```python
from build123d import *

# Parameters (mm, degrees)
ESQUISSE1_R                  = 5
ESQUISSE1_R_2                = 4
BOSS_EXTRU_1_DEPTH           = 15
BOSS_EXTRU_2_START           = 1.5
ESQUISSE2_R                  = 11
ESQUISSE2_R_2                = 5
BOSS_EXTRU_2_DEPTH           = 3.5
ESQUISSE3_R                  = 2
ENL_V_MAT_EXTRU_1_DEPTH      = 22.610182785
R_P_TITION_CIRCULAIRE1_COUNT = 4


with BuildPart() as part:
    # Esquisse1 → Boss.-Extru.1 (new body)
    with BuildSketch(Plane.XY):
        Circle(ESQUISSE1_R)
        Circle(ESQUISSE1_R_2, mode=Mode.SUBTRACT)
    extrude(amount=BOSS_EXTRU_1_DEPTH)

    # Esquisse2 → Boss.-Extru.2 (add)
    with BuildSketch(Plane.XY.offset(BOSS_EXTRU_2_START)):
        Circle(ESQUISSE2_R)
        Circle(ESQUISSE2_R_2, mode=Mode.SUBTRACT)
    extrude(amount=BOSS_EXTRU_2_DEPTH)

    # Esquisse3 → Enlèv. mat.-Extru.1 (cut, through all)
    with BuildSketch(Plane.XY):
        with Locations((0, 8)):
            Circle(ESQUISSE3_R)
    enl_v_mat_extru_1 = extrude(amount=ENL_V_MAT_EXTRU_1_DEPTH, mode=Mode.SUBTRACT)

    # Répétition circulaire1: Enlèv. mat.-Extru.1 ×4 about axis
    r_p_tition_circulaire1_axis = Axis((0, 0, 0), (0, 0, 1))
    for i in range(1, R_P_TITION_CIRCULAIRE1_COUNT):
        add(enl_v_mat_extru_1.rotate(r_p_tition_circulaire1_axis, i * 360 / R_P_TITION_CIRCULAIRE1_COUNT), mode=Mode.SUBTRACT)


solid = part.part
```
Geometry: final body of the model. Coordinates: model frame, mm. A direction names the side the tool comes from. Give positions to 0.01 mm unless a question says otherwise; leave off trailing zeros. Order: outer loops, then holes, each group sorted by start corner. A loop starts at its lowest first (then second) coordinate and runs counter-clockwise, first axis right, second up. Notation, with made-up numbers: (-28.5, -11) -> (5.5, -11) arc R18 cw to (5.5, 6) -> close; hole circle Ø8 at (-9, -34). An arc over 180 degrees is marked (long way). Write each question's results on one line, items separated by ' | '. Start each with the question number.
1) Section D-D (y = 6.5). Return loops of the section in (x, z).
2) Section A-A (y = 0). Return loops of the section in (x, z).
3) Section C-C (z = 3.5). Return loops of the section in (x, y).
4) Set-up query: faces 1 (the cylindrical face through (0, -10, 3)), 2 (the cylindrical face through (-1.08, -4.88, 9.93)), 3 (the flat face through (5, -2, 1.5)). Return all of +Z, -Z, +X, -X, +Y, -Y with unobstructed straight access to the full face (end or side cutting, diameter ignored); none if empty.
5) Draft query along Y for faces 4 (the flat face through (5, -2, 5)), 5 (the cylindrical face through (-1.08, -4.88, 0.74)), 6 (the cylindrical face through (10, 0, 3)). Return one class per face: pulls with the +Y half, pulls with the -Y half, needs draft (parallel to the pull), parting line crosses it, or undercut.
6) First-contact query: pin 1 (8 mm diameter, centred on y = -3.5, z = 10.5, fed in from +X); pin 2 (4 mm diameter, centred on x = 5, z = 9.5, fed in from +Y); pin 3 (4.5 mm diameter, centred on x = 8, y = 0, fed in from +Z). Flat tips, straight axial feed; report the tip coordinate or a pass-through.
7) Line query: line 1 (Y direction, x = 0, z = 3.9); line 2 (X direction, y = -1, z = 1.75); line 3 (Z direction, x = 2.5, y = 9.25). Output: solid intervals per line, ascending. Write a range as from..to.
Calculated:
1) outline: (-8.87, 1.5) -> (-1.32, 1.5) -> (-1.32, 5) -> (-8.87, 5) -> close; (1.32, 1.5) -> (8.87, 1.5) -> (8.87, 5) -> (1.32, 5) -> close
2) outline: (-11, 1.5) -> (-10, 1.5) -> (-10, 5) -> (-11, 5) -> close; (-6, 1.5) -> (-5, 1.5) -> (-5, 0) -> (-4, 0) -> (-4, 15) -> (-5, 15) -> (-5, 5) -> (-6, 5) -> close; (4, 0) -> (5, 0) -> (5, 1.5) -> (6, 1.5) -> (6, 5) -> (5, 5) -> (5, 15) -> (4, 15) -> close; (10, 1.5) -> (11, 1.5) -> (11, 5) -> (10, 5) -> close
3) outline: circle Ø22 at (0, 0); hole circle Ø4 at (-8, 0); hole circle Ø8 at (0, 0); hole circle Ø4 at (0, -8); hole circle Ø4 at (0, 8); hole circle Ø4 at (8, 0)
4) face 1: +Z, -Z | face 2: +Z | face 3: -Z
5) face 4: needs draft | face 5: parting line crosses it | face 6: undercut
6) pin 1: x = 5 | pin 2: y = 4 | pin 3: z = 5
7) line 1: -11..-10, -6..-4, 4..6, 10..11 | line 2: -10.95..-9.73, -6.27..-3.87, 3.87..6.27, 9.73..10.95 | line 3: 1.5..5
